from build123d import *

# Parameters (mm, degrees)
SKETCH1_W               = 75
SKETCH1_H               = 75
BOSS_EXTRUDE1_DEPTH     = 24
SKETCH2_W               = 20
SKETCH2_H               = 19
CUT_EXTRUDE1_DEPTH      = 45
SKETCH3_W               = 19
SKETCH3_H               = 20
CUT_EXTRUDE2_DEPTH      = 45
CUT_EXTRUDE3_DEPTH      = 109.747413762
CUT_EXTRUDE3_DEPTH_BACK = 109.747413762
SKETCH4_W               = 45
SKETCH4_H               = 45
FILLET1_R               = 5
CHAMFER1_SIZE           = 10
SKETCH5_W               = 29
SKETCH5_H               = 15
BOSS_EXTRUDE2_DEPTH     = 37.5
SKETCH6_R               = 11.2
CUT_EXTRUDE4_DEPTH      = 14
FILLET2_R               = 5
CHAMFER3_SIZE           = 5
CUT_EXTRUDE5_DEPTH      = 93.146622293
CUT_EXTRUDE5_DEPTH_BACK = 93.146622293
SKETCH7_R               = 2.65
CUT_EXTRUDE6_DEPTH      = 105.986903945
CUT_EXTRUDE6_DEPTH_BACK = 105.986903945
SKETCH8_R               = 2.65
SKETCH9_R               = 2.65
CUT_EXTRUDE7_DEPTH      = 10
SKETCH10_R              = 2.65
CUT_EXTRUDE8_DEPTH      = 10
CUT_EXTRUDE12_DEPTH     = 19
CUT_EXTRUDE13_REACH     = 111.959
CUT_EXTRUDE14_REACH     = 140.283
SKETCH14_R              = 10
CUT_EXTRUDE15_DEPTH     = 10
CHAMFER5_SIZE           = 4
CHAMFER6_SIZE           = 1
CHAMFER8_SIZE           = 15
CHAMFER8_SIZE_2         = 0.23563883


# Some blends are built 0.0001 mm under size
with BuildPart() as part:
    # Sketch1 → Boss-Extrude1 (new body)
    with BuildSketch(Plane.XY):
        with Locations((37.5, 37.5)):
            Rectangle(SKETCH1_W, SKETCH1_H)
    extrude(amount=BOSS_EXTRUDE1_DEPTH)

    # Sketch2 → Cut-Extrude1 (cut)
    with BuildSketch(Plane.XZ):
        with Locations((15, 14.5)):
            Rectangle(SKETCH2_W, SKETCH2_H)
    extrude(amount=-CUT_EXTRUDE1_DEPTH, mode=Mode.SUBTRACT)

    # Sketch3 → Cut-Extrude2 (cut)
    with BuildSketch(Plane(origin=(75, 0, 0), x_dir=(0, 0, -1), z_dir=(1, 0, 0))):
        with Locations((-14.5, 60)):
            Rectangle(SKETCH3_W, SKETCH3_H)
    extrude(amount=-CUT_EXTRUDE2_DEPTH, mode=Mode.SUBTRACT)

    # Sketch4 → Cut-Extrude3 (cut, two sides: drawn at the far end of the back side and taken through both)
    with BuildSketch(Plane.XY.offset(24).offset(-CUT_EXTRUDE3_DEPTH_BACK)):
        with Locations((52.5, 22.5)):
            Rectangle(SKETCH4_W, SKETCH4_H)
    extrude(amount=CUT_EXTRUDE3_DEPTH + CUT_EXTRUDE3_DEPTH_BACK, mode=Mode.SUBTRACT)

    # Fillet1
    fillet1_edges = [part.edges().sort_by_distance(p)[0] for p in [
        (0, 75, 12),
    ]]
    fillet(fillet1_edges, radius=FILLET1_R)

    # Chamfer1
    chamfer1_edges = [part.edges().sort_by_distance(p)[0] for p in [
        (30, 45, 12),
    ]]
    chamfer(chamfer1_edges, length=CHAMFER1_SIZE)

    # Sketch5 → Boss-Extrude2 (add)
    with BuildSketch(Plane.ZY):
        with Locations((14.5, 36)):
            Rectangle(SKETCH5_W, SKETCH5_H)
    extrude(amount=BOSS_EXTRUDE2_DEPTH)

    # Sketch6 → Cut-Extrude4 (cut)
    with BuildSketch(Plane(origin=(0, 43.5, 0), x_dir=(1, 0, 0), z_dir=(0, 1, 0))):
        with Locations(Location((-21, -15.000000001, 0), (0, 0, 180))):
            Circle(SKETCH6_R)
    extrude(amount=-CUT_EXTRUDE4_DEPTH, mode=Mode.SUBTRACT)

    # Fillet2
    fillet2_edges = [part.edges().sort_by_distance(p)[0] for p in [
        (-37.5, 36, 29),
        (-37.5, 36, 0),
    ]]
    fillet(fillet2_edges, radius=FILLET2_R)

    # Chamfer3
    chamfer3_edges = [part.edges().sort_by_distance(p)[0] for p in [
        (0, 43.5, 12),
        (0, 28.5, 12),
    ]]
    chamfer(chamfer3_edges, length=CHAMFER3_SIZE)

    # Sketch7 → Cut-Extrude5 (cut, two sides: drawn at the far end of the back side and taken through both)
    with BuildSketch(Plane.XZ.offset(-45).offset(-CUT_EXTRUDE5_DEPTH_BACK)):
        with Locations((59, 15)):
            Circle(SKETCH7_R)
    extrude(amount=CUT_EXTRUDE5_DEPTH + CUT_EXTRUDE5_DEPTH_BACK, mode=Mode.SUBTRACT)

    # Sketch8 → Cut-Extrude6 (cut, two sides: drawn at the far end of the back side and taken through both)
    with BuildSketch(Plane(origin=(30, 0, 0), x_dir=(0, 0, -1), z_dir=(1, 0, 0)).offset(-CUT_EXTRUDE6_DEPTH_BACK)):
        with Locations((-15, 16)):
            Circle(SKETCH8_R)
    extrude(amount=CUT_EXTRUDE6_DEPTH + CUT_EXTRUDE6_DEPTH_BACK, mode=Mode.SUBTRACT)

    # Sketch9 → Cut-Extrude7 (cut)
    with BuildSketch(Plane.XY.offset(5)):
        with Locations((15, 22.5)):
            Circle(SKETCH9_R)
    extrude(amount=-CUT_EXTRUDE7_DEPTH, mode=Mode.SUBTRACT)

    # Sketch10 → Cut-Extrude8 (cut)
    with BuildSketch(Plane.XY.offset(5)):
        with Locations((52.5, 60)):
            Circle(SKETCH10_R)
    extrude(amount=-CUT_EXTRUDE8_DEPTH, mode=Mode.SUBTRACT)

    # Sketch11 → Cut-Extrude12 (cut)
    with BuildSketch(Plane.XY.offset(24)):
        Polygon((34, 70), (30, 71), (30, 70), align=None)
        Polygon((30, 50), (34, 50), (30, 49), align=None)
        Polygon((26, 45), (25, 41), (25, 45), align=None)
        Polygon((5, 45), (4, 45), (5, 41), align=None)
    extrude(amount=-CUT_EXTRUDE12_DEPTH, mode=Mode.SUBTRACT)

    # Cut-Extrude13: up to this face of the body (flat: up to its plane)
    cut_extrude13_end = Plane(part.part.faces().sort_by_distance((15, 45, 14.5))[0])
    # Sketch12 → Cut-Extrude13 (cut, up to the picked face)
    with BuildSketch(Plane.XZ, mode=Mode.PRIVATE) as cut_extrude13_sk1:
        Polygon((5, 5), (4, 5), (5, 9), align=None)
    cut_extrude13_tool1 = split(extrude(cut_extrude13_sk1.sketch, amount=-CUT_EXTRUDE13_REACH, mode=Mode.PRIVATE), bisect_by=cut_extrude13_end, keep=Keep.BOTH, mode=Mode.PRIVATE)
    # Sketch12 → Cut-Extrude13 (cut, up to the picked face)
    with BuildSketch(Plane.XZ, mode=Mode.PRIVATE) as cut_extrude13_sk2:
        Polygon((25, 5), (26, 5), (25, 9), align=None)
    cut_extrude13_tool2 = split(extrude(cut_extrude13_sk2.sketch, amount=-CUT_EXTRUDE13_REACH, mode=Mode.PRIVATE), bisect_by=cut_extrude13_end, keep=Keep.BOTH, mode=Mode.PRIVATE)
    add(cut_extrude13_tool1.solids().sort_by(Axis((4.666667, 0, 6.333333), (0, 1, 0)))[0], mode=Mode.SUBTRACT)
    add(cut_extrude13_tool2.solids().sort_by(Axis((25.333333, 0, 6.333333), (0, 1, 0)))[0], mode=Mode.SUBTRACT)

    # Cut-Extrude14: up to this face of the body (flat: up to its plane)
    cut_extrude14_end = Plane(part.part.faces().sort_by_distance((30, 60, 14.5))[0])
    # Sketch13 → Cut-Extrude14 (cut, up to the picked face)
    with BuildSketch(Plane(origin=(75, 0, 0), x_dir=(0, 0, -1), z_dir=(1, 0, 0)), mode=Mode.PRIVATE) as cut_extrude14_sk1:
        Polygon((-5, 50), (-5, 49), (-9, 50), align=None)
    cut_extrude14_tool1 = split(extrude(cut_extrude14_sk1.sketch, amount=-CUT_EXTRUDE14_REACH, mode=Mode.PRIVATE), bisect_by=cut_extrude14_end, keep=Keep.BOTH, mode=Mode.PRIVATE)
    # Sketch13 → Cut-Extrude14 (cut, up to the picked face)
    with BuildSketch(Plane(origin=(75, 0, 0), x_dir=(0, 0, -1), z_dir=(1, 0, 0)), mode=Mode.PRIVATE) as cut_extrude14_sk2:
        Polygon((-5, 70), (-5, 71), (-9, 70), align=None)
    cut_extrude14_tool2 = split(extrude(cut_extrude14_sk2.sketch, amount=-CUT_EXTRUDE14_REACH, mode=Mode.PRIVATE), bisect_by=cut_extrude14_end, keep=Keep.BOTH, mode=Mode.PRIVATE)
    add(cut_extrude14_tool1.solids().sort_by(Axis((75, 49.666667, 6.333333), (-1, 0, 0)))[0], mode=Mode.SUBTRACT)
    add(cut_extrude14_tool2.solids().sort_by(Axis((75, 70.333333, 6.333333), (-1, 0, 0)))[0], mode=Mode.SUBTRACT)

    # Sketch14 → Cut-Extrude15 (cut)
    with BuildSketch(Plane(origin=(0, 29.5, 0), x_dir=(1, 0, 0), z_dir=(0, 1, 0))):
        with Locations(Location((-21, -15.000000001, 0), (0, 0, 180))):
            Circle(SKETCH14_R)
    extrude(amount=-CUT_EXTRUDE15_DEPTH, mode=Mode.SUBTRACT)

    # Chamfer5
    chamfer5_edges = [part.edges().sort_by_distance(p)[0] for p in [
        (0, 36, 24),
    ]]
    chamfer(chamfer5_edges, length=CHAMFER5_SIZE)

    # Chamfer6
    chamfer6_edges = [part.edges().sort_by_distance(p)[0] for p in [
        (0, 36, 29),
    ]]
    chamfer(chamfer6_edges, length=CHAMFER6_SIZE - 0.0001)  # a hair under: the kernel refuses the full size

    # Chamfer8
    # the kernel refuses this chamfer: 15, 0.23563883 mm, written as the material it adds along each edge
    with BuildSketch(Plane(origin=(-21, 29.5, 15.000000001), x_dir=(-1, 0, 0), z_dir=(0, 0, -1))) as chamfer8_piece_1_section:
        Polygon((11.2, CHAMFER8_SIZE), (11.2 - CHAMFER8_SIZE_2, 0), (11.2, 0), align=None)
    chamfer8_piece_1 = revolve(axis=Axis((-21, 29.5, 15.000000001), (0, 1, 0)), mode=Mode.PRIVATE)
    chamfer8_piece_1 = split(chamfer8_piece_1, bisect_by=Plane(origin=(-9.855053723, 43.5, 15.000000001), z_dir=(0, -1, 0)), keep=Keep.TOP, mode=Mode.PRIVATE)
    add(chamfer8_piece_1)


solid = part.part
CAD build for the part. Positions are in the model's coordinates, mm. A direction names the side the tool comes from. Round coordinates to 2 decimals unless told otherwise and drop trailing zeros. Order: outer loops, then holes, each group sorted by start corner. A loop starts at its lowest first (then second) coordinate and runs counter-clockwise, first axis right, second up. Notation, with made-up numbers: M 84.25,-5 L 105.25,-5 A36 ccw 105.25,31 Z; hole C 19,33.25 d1. An arc over 180 degrees is marked long. Use one line per item in the form item = value.
Q1. Flat gauge pins, fed straight in: P1, Ø2, axis at y = 57, z = 16, coming from the +X side; P2, Ø6.5, axis at y = 63.5, z = 14, coming from the -X side; P3, Ø6.5, axis at x = 59.5, y = 62, coming from the +Z side. Where does each tip first touch, or does it go through?
Recorded:
P1 = 30
P2 = 0
P3 = 5
Q2. Probe L1, parallel to Y at x = 51.5, z = 11; L2, parallel to Z at x = 59, y = 73.6; L3, parallel to Y at x = 52.5, z = 1.35. List the from-to ranges inside material, lowest first.
Recorded:
L1 = 45 to 50, 70 to 75
L2 = 0 to 12.35, 17.65 to 24
L3 = 45 to 57.35, 62.65 to 75
Q3. Which spindle directions (+Z, -Z, +X, -X, +Y, -Y) get a long thin tool onto all of the face, cutting with end or side? Do faces 5 (the flat face through (5, 20, 16)), 6 (the flat face through (25.5, 43, 14.6)), 7 (the flat face through (25.5, 22.2, 7)), 8 (the flat face through (55, 50, 17)). Say none if no direction does.
Recorded:
face_5 = +Z, -Y
face_6 = +Z
face_7 = -Y
face_8 = +Z, +X
Q4. Saw through at D-D on z = 15. State how many separate pieces and enclosed holes the cut face has, then the cut area to 3 significant figures.
Recorded:
separate_pieces = 6
enclosed_holes = 0
area = 1,990 mm^2
Q5. Two-plate mould, pull along X, no slides. Class faces 1 (the flat face through (35, 40, 12)), 2 (the cylindrical face through (61.45, 47.54, 13.99)), 3 (the flat face through (22, 45, 0)), 4 (the flat face through (20, 22, 5)): +X half, -X half, draft (parallel to the pull), parting line (faces both ways), or undercut.
Recorded:
face_1 = +X half
face_2 = undercut
face_3 = draft
face_4 = undercut
Q6. Saw through at A-A on y = 60. Give the cut face in (x, z), then the cut area to 4 significant figures.
Recorded:
outline = M 0,0 L 49.85,0 L 49.85,5 L 30,5 L 30,24 L 0,24 Z; M 55.15,0 L 75,0 L 75,5 L 55.15,5 Z
area = 918.5 mm^2
Q7. Saw through at B-B on x = 52.5. Give the cut face in (y, z).
Recorded:
outline = M 45,0 L 57.35,0 L 57.35,5 L 49,5 L 50,9 L 50,24 L 45,24 Z; M 62.65,0 L 75,0 L 75,24 L 70,24 L 70,9 L 71,5 L 62.65,5 Z
Q8. Saw through at C-C on y = 16. Give the cut face in (x, z).
Recorded:
outline = M 0,0 L 30,0 L 30,12.35 L 25,12.35 L 25,9 L 26,5 L 4,5 L 5,9 L 5,12.35 L 0,12.35 Z; M 0,17.65 L 5,17.65 L 5,24 L 0,24 Z; M 25,17.65 L 30,17.65 L 30,24 L 25,24 Z
